from build123d import *

# Parameters (mm, degrees)
SZKIC1_W                    = 70
SZKIC1_H                    = 85.85
DODANIE_WYCI_GNI_CIE1_DEPTH = 15
SZKIC2_R                    = 3
WYTNIJ_WYCI_GNI_CIE1_DEPTH  = 15
SZKIC3_R                    = 5
WYTNIJ_WYCI_GNI_CIE2_DEPTH  = 7
SZKIC4_R                    = 3
WYTNIJ_WYCI_GNI_CIE3_DEPTH  = 15
SZYK_LINIOWY1_COUNT         = 2
SZYK_LINIOWY1_PITCH         = 55
SZYK_LINIOWY1_COUNT_DIR2    = 2
SZYK_LINIOWY1_PITCH_DIR2    = 70.85


with BuildPart() as part:
    # Szkic1 → Dodanie-wyciągnięcie1 (new body)
    with BuildSketch(Plane.XY):
        Rectangle(SZKIC1_W, SZKIC1_H)
    extrude(amount=DODANIE_WYCI_GNI_CIE1_DEPTH)

    # Szkic2 → Wytnij-wyciągnięcie1 (cut)
    with BuildSketch(Plane.XY.offset(15)):
        with Locations((-13.5, 34.925)):
            Circle(SZKIC2_R)
        with Locations((-13.5, -34.925)):
            Circle(SZKIC2_R)
    extrude(amount=-WYTNIJ_WYCI_GNI_CIE1_DEPTH, mode=Mode.SUBTRACT)

    # Szkic3 → Wytnij-wyciągnięcie2 (cut)
    with BuildSketch(Plane.XY.offset(15)):
        with Locations((-13.5, 34.925)):
            Circle(SZKIC3_R)
        with Locations((-13.5, -34.925)):
            Circle(SZKIC3_R)
    extrude(amount=-WYTNIJ_WYCI_GNI_CIE2_DEPTH, mode=Mode.SUBTRACT)

    # Szkic4 → Wytnij-wyciągnięcie3 (cut)
    with BuildSketch(Plane.XY.offset(15)):
        with Locations((27.5, 35.425)):
            Circle(SZKIC4_R)
    wytnij_wyci_gni_cie3 = extrude(amount=-WYTNIJ_WYCI_GNI_CIE3_DEPTH, mode=Mode.SUBTRACT)

    # Szyk liniowy1: Wytnij-wyci_gni_cie3 2 × 2
    with Locations(*[(-i * SZYK_LINIOWY1_PITCH, -j * SZYK_LINIOWY1_PITCH_DIR2, 0) for i in range(SZYK_LINIOWY1_COUNT) for j in range(SZYK_LINIOWY1_COUNT_DIR2) if (i, j) != (0, 0)]):
        add(wytnij_wyci_gni_cie3, mode=Mode.SUBTRACT)


solid = part.part
Check sheet for the modelled part. Datum: model origin and axes. Units: mm. A direction names the side the tool comes from. Coordinates: 2 decimals unless noted, no trailing zeros. Loops run counter-clockwise (first coordinate to the right, second up) from the corner with the lowest first, then second, coordinate; pieces in that order, holes last. Notation, with made-up numbers: (8.25, 86) -> (61.25, 86) arc R25 cw to (61.25, 107) -> close; hole circle Ø7 at (1.5, 37.25). An arc over 180 degrees is marked (long way). Write item = value, one per line. Start each with the question number.
1. Section check A-A on x = -27.5. Record the cut outline in (y, z) (3 decimals), then the cut area to 3 significant figures.
2. Section check B-B on z = 6.5. Record the cut outline in (x, y) (3 decimals).
3. Section check C-C on x = -13.5. Record the cut outline in (y, z) (3 decimals).
4. Draft check along X on faces 1 (the flat face through (-35, -1, 7)), 2 (the flat face through (0, -42.925, 7)), 3 (the flat face through (35, -1, 7)), 4 (the flat face through (-11, -37, 8)). Enter one of: released by +X, released by -X, zero draft, split by the parting line, or undercut.
5. Section check D-D on x = 28. Record the cut outline in (y, z) (3 decimals), then the cut area to 3 significant figures.
6. Depth check by flat-ended pin: P1, Ø5.5, axis at x = -13.5, y = 34.925, coming from the +Z side (1 decimal); P2, Ø3, axis at x = -13.5, y = -36.5, coming from the +Z side. Enter the tip coordinate at first touch or a pass-through.
7. Material ranges on line 1 (Y direction, x = 27.5, z = 9.75) (3 decimals); line 2 (Y direction, x = -13.5, z = 4.5) (3 decimals); line 3 (X direction, y = 36.5, z = 3.75), recorded low to high.
8. Tool access check on faces 5 (the cylindrical face through (-10.81, -30.71, 11.55)), 6 (the cylindrical face through (-15.711, 36.953, 4.056)). Record the directions out of +Z, -Z, +X, -X, +Y, -Y that give a thin tool (end or side, any length) a straight path to the whole face; none if there is none.
Responses:
q1.outline = (-42.925, 0) -> (-38.425, 0) -> (-38.425, 15) -> (-42.925, 15) -> close; (-32.425, 0) -> (32.425, 0) -> (32.425, 15) -> (-32.425, 15) -> close; (38.425, 0) -> (42.925, 0) -> (42.925, 15) -> (38.425, 15) -> close
q1.area = 1,110 mm2
q2.outline = (-35, -42.925) -> (35, -42.925) -> (35, 42.925) -> (-35, 42.925) -> close; hole circle Ø6 at (-27.5, -35.425); hole circle Ø6 at (-27.5, 35.425); hole circle Ø6 at (-13.5, -34.925); hole circle Ø6 at (-13.5, 34.925); hole circle Ø6 at (27.5, -35.425); hole circle Ø6 at (27.5, 35.425)
q3.outline = (-42.925, 0) -> (-37.925, 0) -> (-37.925, 8) -> (-39.925, 8) -> (-39.925, 15) -> (-42.925, 15) -> close; (-31.925, 0) -> (31.925, 0) -> (31.925, 8) -> (29.925, 8) -> (29.925, 15) -> (-29.925, 15) -> (-29.925, 8) -> (-31.925, 8) -> close; (37.925, 0) -> (42.925, 0) -> (42.925, 15) -> (39.925, 15) -> (39.925, 8) -> (37.925, 8) -> close
q4.face_1 = released by -X
q4.face_2 = zero draft
q4.face_3 = released by +X
q4.face_4 = undercut
q5.outline = (-42.925, 0) -> (-38.383, 0) -> (-38.383, 15) -> (-42.925, 15) -> close; (-32.467, 0) -> (32.467, 0) -> (32.467, 15) -> (-32.467, 15) -> close; (38.383, 0) -> (42.925, 0) -> (42.925, 15) -> (38.383, 15) -> close
q5.area = 1,110 mm2
q6.P1 = through
q6.P2 = 8
q7.line_1 = -42.925 to -38.425, -32.425 to 32.425, 38.425 to 42.925
q7.line_2 = -42.925 to -37.925, -31.925 to 31.925, 37.925 to 42.925
q7.line_3 = -35 to -30.3, -24.7 to -16.05, -10.95 to 24.7, 30.3 to 35
q8.face_5 = +Z
q8.face_6 = +Z, -Z
